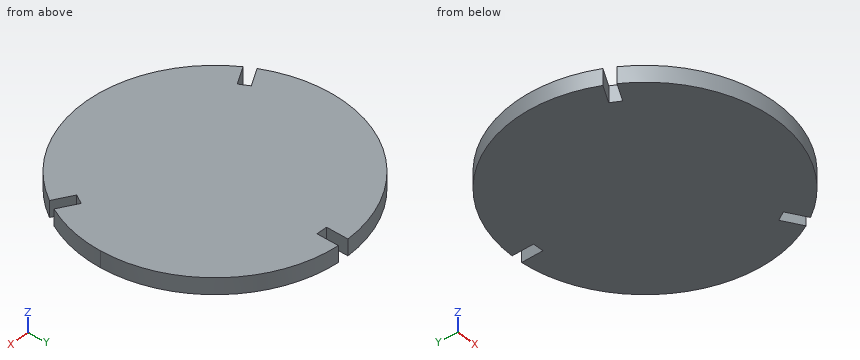
```python
from build123d import *

# Parameters (mm, degrees)
F1_DEPTH = 19.05


with BuildPart() as f1:
    # F0 (on Top) → F1 (new body)
    with BuildSketch(Plane.XY):
        with BuildLine():
            ThreePointArc((135.042654, -70.634564), (147.997062, -36.367977), (152.4, 0))
            ThreePointArc((152.4, 0), (109.985226, 105.494123), (6.35, 152.267651))
            Line((6.35, 152.267651), (6.35, 126.867651))
            Line((6.35, 126.867651), (-6.35, 126.867651))
            Line((-6.35, 126.867651), (-6.35, 152.267651))
            ThreePointArc((-6.35, 152.267651), (-131.982272, 76.2), (-135.042654, -70.634564))
            Line((-135.042654, -70.634564), (-113.045609, -57.934564))
            Line((-113.045609, -57.934564), (-106.695609, -68.933087))
            Line((-106.695609, -68.933087), (-128.692654, -81.633087))
            ThreePointArc((-128.692654, -81.633087), (0, -152.4), (128.692654, -81.633087))
            Line((128.692654, -81.633087), (106.695609, -68.933087))
            Line((106.695609, -68.933087), (113.045609, -57.934564))
            Line((113.045609, -57.934564), (135.042654, -70.634564))
        make_face()
    extrude(amount=F1_DEPTH)


solid = f1.part
```
Check sheet for the modelled part. Datum: model origin and axes. Units: mm. Round coordinates to 2 decimals unless told otherwise and drop trailing zeros. Order: outer loops, then holes, each group sorted by start corner. A loop starts at its lowest first (then second) coordinate and runs counter-clockwise, first axis right, second up.
1) Section check C-C (y = 90). Record the boundary of the cut face in (x, z).
2) Section check A-A (z = 15.25). Record the boundary of the cut face in (x, y), and give its area (3 significant figures).
3) Go/stop test with flat-tipped pins: pin 1 Ø10 at (x, z) = (-0.5, 12) entering from +Y; pin 2 Ø1 at (x, z) = (113, 3.5) entering from -Y; pin 3 Ø6 at (x, z) = (65.5, 13) entering from +Y. Record where each tip stops, or that it passes through.
4) Section check D-D (x = 55). Record the boundary of the cut face in (y, z), and give its area (3 significant figures).
5) Scan lines: line 1 (Y direction, x = 119.5, z = 13); line 2 (X direction, y = 139, z = 12.25); line 3 (Y direction, x = -98.5, z = 5). Record each from-to range of solid material in increasing order.
6) Section check B-B (x = 117.5). Record the boundary of the cut face in (y, z), and give its area (3 significant figures).
Result:
1. outline: (-122.99, 0) - (122.99, 0) - (122.99, 19.05) - (-122.99, 19.05) - close
2. outline: (-135.04, -70.63) - (-113.05, -57.93) - (-106.7, -68.93) - (-128.69, -81.63) arc R152.4 ccw to (128.69, -81.63) - (106.7, -68.93) - (113.05, -57.93) - (135.04, -70.63) arc R152.4 ccw to (152.4, 0) arc R152.4 ccw to (6.35, 152.27) - (6.35, 126.87) - (-6.35, 126.87) - (-6.35, 152.27) arc R152.4 ccw to start
2. area: 72,000 mm2
3. pin 1: stops at y = 126.87
3. pin 2: stops at y = -102.81
3. pin 3: stops at y = 138.99
4. outline: (-142.13, 0) - (142.13, 0) - (142.13, 19.05) - (-142.13, 19.05) - close
4. area: 5,420 mm2
5. line 1: y = -94.58 to -76.33, -61.66 to 94.58
5. line 2: x = -62.49 to -6.35, 6.35 to 62.49
5. line 3: y = -116.29 to 116.29
6. outline: (-97.05, 0) - (-75.17, 0) - (-75.17, 19.05) - (-97.05, 19.05) - close; (-60.51, 0) - (97.05, 0) - (97.05, 19.05) - (-60.51, 19.05) - close
6. area: 3,420 mm2
